```python
from build123d import *

# Parameters (mm, degrees)
SKETCH4_W               = 2.032
SKETCH4_H               = 2.54
SKETCH5_R               = 76.2
SKETCH5_R_2             = 31.75
BOSS_EXTRUDE1_DEPTH     = 3.81
SKETCH6_R               = 76.2
SKETCH6_R_2             = 62.23
BOSS_EXTRUDE2_DEPTH     = 10.16
CUT_EXTRUDE1_DEPTH      = 113.342968182
CUT_EXTRUDE1_DEPTH_BACK = 113.342968182
SKETCH2_R               = 6.35
SKETCH3_R               = 3.175
CUT_EXTRUDE2_DEPTH      = 113.342968182
CIRPATTERN1_COUNT       = 8


with BuildPart() as part:
    # Sketch1 → Revolve1 (revolve)
    with BuildSketch(Plane.XY, mode=Mode.PRIVATE) as revolve1_sk:
        with BuildLine():
            Line((0, 76.2), (-10.16, 76.2))
            Line((-10.16, 76.2), (-10.16, 21.082))
            ThreePointArc((-10.16, 21.082), (-11.647897552, 17.489897552), (-15.24, 16.002))
            Line((-15.24, 16.002), (-31.75, 16.002))
            Line((-31.75, 16.002), (-31.75, 9.652))
            Line((-31.75, 9.652), (-6.35, 9.652))
            Line((-6.35, 9.652), (-6.35, 19.812))
            ThreePointArc((-6.35, 19.812), (-5.606051224, 21.608051224), (-3.81, 22.352))
            Line((-3.81, 22.352), (0, 22.352))
            Line((0, 22.352), (0, 76.2))
        make_face()
    revolve(revolve1_sk.sketch.rotate(Axis((0, 0, 0), (-1, 0, 0)), 90), axis=Axis((0, 0, 0), (-1, 0, 0)))

    # Sketch4 → Cut-Revolve1 (revolve, cut)
    with BuildSketch(Plane.XY):
        with Locations((-1.016, 24.892)):
            Rectangle(SKETCH4_W, SKETCH4_H)
    revolve(axis=Axis((0, 0, 0), (-1, 0, 0)), mode=Mode.SUBTRACT)

    # Sketch5 → Boss-Extrude1 (add)
    with BuildSketch(Plane(origin=(0, 0, 0), x_dir=(0, 0, -1), z_dir=(1, 0, 0))):
        Circle(SKETCH5_R)
        with Locations(Location((0, 0, 0), (0, 0, 180))):
            Circle(SKETCH5_R_2, mode=Mode.SUBTRACT)
    extrude(amount=BOSS_EXTRUDE1_DEPTH)

    # Sketch6 → Boss-Extrude2 (add)
    with BuildSketch(Plane(origin=(3.81, 0, 0), x_dir=(0, 0, -1), z_dir=(1, 0, 0))):
        Circle(SKETCH6_R)
        Circle(SKETCH6_R_2, mode=Mode.SUBTRACT)
    extrude(amount=BOSS_EXTRUDE2_DEPTH)

    # Sketch2 → Cut-Extrude1 (cut, two sides: drawn at the far end of the back side and taken through both)
    with BuildSketch(Plane(origin=(0, 0, 0), x_dir=(0, 0, -1), z_dir=(1, 0, 0)).offset(-CUT_EXTRUDE1_DEPTH_BACK)):
        with Locations((41.275, 0)):
            Circle(SKETCH2_R)
        with Locations((-41.275, 0)):
            Circle(SKETCH2_R)
    extrude(amount=CUT_EXTRUDE1_DEPTH + CUT_EXTRUDE1_DEPTH_BACK, mode=Mode.SUBTRACT)

    # Sketch3 → Cut-Extrude2 (cut, symmetric)
    with BuildSketch(Plane(origin=(0, 0, 0), x_dir=(0, 0, -1), z_dir=(1, 0, 0))):
        with Locations(Location((64.77, 0, 0), (0, 0, 216.018854193))):
            Circle(SKETCH3_R)
    cut_extrude2 = extrude(amount=CUT_EXTRUDE2_DEPTH, both=True, mode=Mode.SUBTRACT)

    # CirPattern1: Cut-Extrude2 ×8 about axis
    cirpattern1_axis = Axis((0, 0, 0), (1, 0, 0))
    for i in range(1, CIRPATTERN1_COUNT):
        add(cut_extrude2.rotate(cirpattern1_axis, i * 360 / CIRPATTERN1_COUNT), mode=Mode.SUBTRACT)


solid = part.part
```
Geometry check sheet. Reference: the model listing, model coordinates, mm. A direction names the side the tool comes from. Round coordinates to 2 decimals unless told otherwise and drop trailing zeros. Order: outer loops, then holes, each group sorted by start corner. A loop starts at its lowest first (then second) coordinate and runs counter-clockwise, first axis right, second up. Notation, with made-up numbers: (54.5, 7) - (84.5, 7) arc R11 ccw to (84.5, 25) - close; hole circle Ø8 at (41.5, 55). An arc over 180 degrees is marked (long way). Use a Markdown table: item, result. Add a question column.
1) Thickness scan on line 1 along Y through (x, z) = (-1.25, 0) (3 decimals); line 2 along Z through (x, y) = (0.5, 4); line 3 along Y through (x, z) = (-18.5, 0). Record the ranges inside material, lowest first.
2) Gauge pin test, flat ends, axial feed: P1, Ø2, axis at y = 26.5, z = -39, coming from the -X side; P2, Ø8, axis at x = -12, y = -5.5, coming from the +Z side; P3, Ø4, axis at x = -16.5, z = -10.5, coming from the +Y side. Record the tip position at first contact, or that the pin passes through.
3) Mould release check, pull along Y, two halves, no side actions. Record for faces 1 (the flat face through (0, 21, 9)), 2 (the flat face through (-10.16, 16, -16)), 3 (the cylindrical face through (1.736, -46.367, 60.47)): released by +Y, released by -Y, zero draft, split by the parting line, or undercut.
4) Section check A-A (z = 64.77). Record the cut outline in (x, y) (3 decimals).
5) Set-up check for faces 4 (the cylindrical face through (2.074, -0.359, -67.925)), 5 (the cylindrical face through (8.819, 23.522, -57.613)): record each of +Z, -Z, +X, -X, +Y, -Y from which the full face is reachable in a straight line by a thin tool's end or side.
6) Section check D-D (y = 39). Record the cut outline in (x, z).
7) Section check C-C (z = 0). Count the separate pieces of the cut face and the enclosed holes in it, then the cut area to 3 significant figures.
Established:
| question | item | result |
|---|---|---|
| 1 | line 1 | -76.2 to -67.945, -61.595 to -26.162, -23.622 to -22.352, 22.352 to 23.622, 26.162 to 61.595, 67.945 to 76.2 |
| 1 | line 2 | -76.09 to -46.21, -36.34 to -31.5, 31.5 to 36.34, 46.21 to 76.09 |
| 1 | line 3 | -16 to -9.65, 9.65 to 16 |
| 2 | P1 | x = -10.16 |
| 2 | P2 | z = 76.18 |
| 2 | P3 | y = 13.56 |
| 3 | face 1 | undercut |
| 3 | face 2 | zero draft |
| 3 | face 3 | split by the parting line |
| 4 | outline | (-10.16, -40.141) - (13.97, -40.141) - (13.97, -3.175) - (-10.16, -3.175) - close; (-10.16, 3.175) - (13.97, 3.175) - (13.97, 40.141) - (-10.16, 40.141) - close |
| 5 | face 4 | +X, -X |
| 5 | face 5 | +X |
| 6 | outline | (-10.16, -65.46) - (13.97, -65.46) - (13.97, -48.49) - (3.81, -48.49) - (3.81, 48.49) - (13.97, 48.49) - (13.97, 65.46) - (-10.16, 65.46) - close |
| 7 | separate pieces | 4 |
| 7 | enclosed holes | 0 |
| 7 | area | 1,800 mm2 |
